Check sheet for the modelled part. Datum: model origin and axes. Units: mm. A direction names the side the tool comes from. Coordinates: 2 decimals unless noted, no trailing zeros. Loops run counter-clockwise (first coordinate to the right, second up) from the corner with the lowest first, then second, coordinate; pieces in that order, holes last. Notation, with made-up numbers: M 22,-7.75 L 50,-7.75 A26 ccw 50,16.25 Z; hole C 58,43 d5. An arc over 180 degrees is marked long. Use CSV: the item, a comma, the result in double quotes. Start each with the question number.
(1) Section check C-C on x = -34. Record the cut outline in (y, z) (3 decimals), and give its area (3 significant figures).
(2) Set-up check for faces 1 (the flat face through (4.689, 9, 6)), 2 (the cylindrical face through (-29.71, 11.68, 6.11)), 3 (the cylindrical face through (-14, -4.14, 6.73)): record each of +Z, -Z, +X, -X, +Y, -Y from which the full face is reachable in a straight line by a thin tool's end or side.
(3) Go/stop test with flat-tipped pins: pin 1 Ø10 at (x, y) = (-27, -6) entering from -Z; pin 2 Ø9.5 at (x, y) = (-14, 8) entering from +Z; pin 3 Ø12 at (x, z) = (0, 2.5) entering from -Y; pin 4 Ø4 at (x, y) = (-24.5, 9.5) entering from -Z (3 decimals). Record where each tip stops, or that it passes through.
(4) Section check A-A on z = 6. Record the cut outline in (x, y), and give its area (3 significant figures).
(5) Scan lines: line 1 (Y direction, x = -10.5, z = 2.25); line 2 (Z direction, x = -27.5, y = 8.75); line 3 (Z direction, x = -14.5, y = 12.5). Record each from-to range of solid material in increasing order.
(6) Draft check along Z on faces 4 (the cylindrical face through (-2.92, 11.57, 6.73)), 5 (the flat face through (-27, 9, 24.99)), 6 (the flat face through (-10.311, 6.5, 5.9)), 7 (the flat face through (-16, 15.258, 6)). Enter one of: pulls with the +Z half, pulls with the -Z half, needs draft (parallel to the pull), parting line crosses it, or undercut.
from build123d import *

# Parameters (mm, degrees)
F0_W     = 12
F0_H     = 12
F1_DEPTH = 12
F2_R     = 2.425
F3_DEPTH = 15
F4_R     = 2.425
F5_DEPTH = 15
F6_R     = 2.425
F7_DEPTH = 15
F8_R     = 2.425


with BuildPart() as f1:
    # F0 (on Top) → F1 (new body)
    with BuildSketch(Plane.XY):
        with Locations((-16.311498, 9.258204)):
            Rectangle(F0_W, F0_H)
    extrude(amount=F1_DEPTH)

    # F2 (on face) → F3 (join)
    with BuildSketch(Plane.YZ.offset(-10.311498)):
        with Locations((9.258204, 6)):
            Circle(F2_R)
    extrude(amount=F3_DEPTH)

    # F4 (on face) → F5 (join)
    with BuildSketch(Plane(origin=(-22.311498, 0, 0), x_dir=(0, -1, 0), z_dir=(-1, 0, 0))):
        with Locations((-9.258204, 6)):
            Circle(F4_R)
    extrude(amount=F5_DEPTH)

    # F6 (on face) → F7 (join)
    with BuildSketch(Plane.XZ.offset(-3.258204)):
        with Locations((-16.311498, 6)):
            Circle(F6_R)
    extrude(amount=F7_DEPTH)

    # F10: sweep along a path in F9
    with BuildLine(Plane(origin=(0, 15.258204, 0), x_dir=(-1, 0, 0), z_dir=(0, 1, 0))) as f10_path:
        Line((12.736498, 12), (5.236498, 24.990381))
    # F8 (on face) → F10 (sweep)
    with BuildSketch(Plane.XY.offset(12)):
        with Locations((-12.736498, 9.258204)):
            Circle(F8_R)
    sweep(path=f10_path.line)

    # F11: sweep along a path in F9
    with BuildLine(Plane(origin=(0, 15.258204, 0), x_dir=(-1, 0, 0), z_dir=(0, 1, 0))) as f11_path:
        Line((19.886498, 12), (27.386498, 24.990381))
    # F8 (on face) → F11 (sweep)
    with BuildSketch(Plane.XY.offset(12)):
        with BuildLine():
            ThreePointArc((-22.311498, 9.258204), (-19.886498, 6.833204), (-17.461498, 9.258204))
            ThreePointArc((-17.461498, 9.258204), (-19.886498, 11.683204), (-22.311498, 9.258204))
        make_face()
    sweep(path=f11_path.line)


solid = f1.part
Outcome:
1,outline,"C 9.258,6 d4.85"
1,area,"18.5 mm²"
2,face 1,"+Z, -Z, +X, +Y, -Y"
2,face 2,"-X"
2,face 3,"-Y"
3,pin 1,"passes through"
3,pin 2,"stops at z = 22.05"
3,pin 3,"stops at y = 6.83"
3,pin 4,"stops at z = 3.575"
4,outline,"M -37.31,6.83 L -22.31,6.83 L -22.31,3.26 L -18.74,3.26 L -18.74,-11.74 L -13.89,-11.74 L -13.89,3.26 L -10.31,3.26 L -10.31,6.83 L 4.69,6.83 L 4.69,11.68 L -10.31,11.68 L -10.31,15.26 L -22.31,15.26 L -22.31,11.68 L -37.31,11.68 Z"
4,area,"362 mm²"
5,line 1,"y = 3.26 to 15.26"
5,line 2,"z = 3.63 to 8.37, 21.08 to 24.99"
5,line 3,"z = 0 to 12"
6,face 4,"undercut"
6,face 5,"pulls with the +Z half"
6,face 6,"undercut"
6,face 7,"needs draft"
